```python
from build123d import *

# Parameters (mm, degrees)
F0_W     = 50.8
F0_H     = 50.8
F1_DEPTH = 7.62
F2_T     = -1.27
F3_W     = 1.27
F3_H     = 43.18
F4_DEPTH = 6.35


with BuildPart() as f1:
    # F0 (on Top) → F1 (new body)
    with BuildSketch(Plane.XY):
        with Locations((-25.4, 25.4)):
            Rectangle(F0_W, F0_H)
    extrude(amount=F1_DEPTH)

    # F2
    f2_openings = [f1.faces().sort_by_distance(p)[0] for p in [
        (-25.4, 25.4, 7.62),
    ]]
    offset(amount=F2_T, openings=f2_openings)

    # F3 (on face) → F4 (join)
    with BuildSketch(Plane.XY.offset(1.27)):
        with Locations((-43.815, 22.86)):
            Rectangle(F3_W, F3_H)
    extrude(amount=F4_DEPTH)


solid = f1.part
```
Here's how the part is built. I have some questions about the finished solid (model axes, mm). A direction names the side the tool comes from. Coordinates: 2 decimals unless noted, no trailing zeros. Order: outer loops, then holes, each group sorted by start corner. A loop starts at its lowest first (then second) coordinate and runs counter-clockwise, first axis right, second up. Notation, with made-up numbers: (-35, -28) -> (17, -28) arc R13 ccw to (17, -13) -> close; hole circle Ø11 at (52.5, 65.25). An arc over 180 degrees is marked (long way). Return JSON: item names as keys, results as strings.
1) On a 3-axis mill with a long thin cutter (end or side, diameter ignored), from which of +Z, -Z, +X, -X, +Y, -Y can I reach the whole of each face in a straight line? I mean faces 4 (the flat face through (-49.53, 25, 4)), 5 (the flat face through (-50.8, 25, 4)). Say none if no direction works.
Conclusion:
{"face 4": "+Z", "face 5": "+Z, -Z, -X, +Y, -Y"}
2) I'm going to push a flat-ended pin straight in: P1, Ø1, axis at x = -26.5, y = 32.5, coming from the +Z side. Where does the tip first touch, or does it pass through?
Conclusion:
{"P1": "stops at z = 1.27"}
3) If we section it at B-B on y = 41: List the corners of the cut face in (x, z) for me, plus the area to 3 significant figures.
Conclusion:
{"outline": "(-50.8, 0) -> (0, 0) -> (0, 7.62) -> (-1.27, 7.62) -> (-1.27, 1.27) -> (-43.18, 1.27) -> (-43.18, 7.62) -> (-44.45, 7.62) -> (-44.45, 1.27) -> (-49.53, 1.27) -> (-49.53, 7.62) -> (-50.8, 7.62) -> close", "area": "88.7 mm²"}
4) Thinking about a two-plate mould opening in X: for faces 1 (the flat face through (-47, 1.27, 4)), 2 (the flat face through (0, 25, 4)), 3 (the flat face through (-26, 0, 4)), which applies, +X half, -X half, draft (parallel to the pull), parting line (faces both ways), or undercut?
Conclusion:
{"face 1": "undercut", "face 2": "+X half", "face 3": "draft"}
5) If I drill on probe 1 along X at (y, z) = (36, 2.5); probe 2 along Y at (x, z) = (-11, 2.25); probe 3 along X at (y, z) = (47, 4.75), over which ranges is the centre line in solid material (lowest first)?
Conclusion:
{"probe 1": "x = -50.8 to -49.53, -44.45 to -43.18, -1.27 to 0", "probe 2": "y = 0 to 1.27, 49.53 to 50.8", "probe 3": "x = -50.8 to -49.53, -1.27 to 0"}
6) If we section it at C-C on x = -23: List the corners of the cut face in (y, z) for me.
Conclusion:
{"outline": "(0, 0) -> (50.8, 0) -> (50.8, 7.62) -> (49.53, 7.62) -> (49.53, 1.27) -> (1.27, 1.27) -> (1.27, 7.62) -> (0, 7.62) -> close"}
7) If we section it at A-A on z = 6.75: List the corners of the cut face in (x, y) for me, plus the area to 3 significant figures.
Conclusion:
{"outline": "(-50.8, 0) -> (0, 0) -> (0, 50.8) -> (-50.8, 50.8) -> close; hole (-49.53, 1.27) -> (-44.45, 1.27) -> (-44.45, 44.45) -> (-43.18, 44.45) -> (-43.18, 1.27) -> (-1.27, 1.27) -> (-1.27, 49.53) -> (-49.53, 49.53) -> close", "area": "306 mm²"}
